Autodesk Inventor part; units mm, degrees
ref_plane "YZ Plane" through (0, 0, 0) normal (1, 0, 0) x (0, 1, 0)
ref_plane "XZ Plane" through (0, 0, 0) normal (0, 1, 0) x (-1, 0, 0)
ref_plane "XY Plane" through (0, 0, 0) normal (0, 0, 1) x (1, 0, 0)
sketch "Skizze1" plane through (0, 0, 0) normal (0, 0, 1) x (1, 0, 0)
  circle A0 centre (0, 0) radius 4.95
  circle A1 centre (-130, 0) radius 4.95
  circle A2 centre (130, 0) radius 4.95
  dimension "d0" = 9.9
  dimension "d1" = 9.9
  dimension "d2" = 130
  dimension "d3" = 9.9
  dimension "d4" = 130
extrude "Extrusion1" add sketch "Skizze1" along normal blind 10
sketch "Skizze2" plane through (0, 0, 0) normal (0, 0, -1) x (-1, 0, 0)
  line L0 (132.5, -10) -> (-132.5, -10)
  line L1 (-140, -2.5) -> (-140, 2.5)
  line L2 (-132.5, 10) -> (132.5, 10)
  line L3 (140, 2.5) -> (140, -2.5)
  arc A0 (132.5, -10) -> (140, -2.5) centre (132.5, -2.5) ccw
  arc A1 (140, 2.5) -> (132.5, 10) centre (132.5, 2.5) ccw
  arc A2 (-132.5, 10) -> (-140, 2.5) centre (-132.5, 2.5) ccw
  arc A3 (-140, -2.5) -> (-132.5, -10) centre (-132.5, -2.5) ccw
  point P0 (0, 0)
  point P1 (140, -10)
  point P2 (-140, -10)
  point P3 (140, 10)
  dimension "d7" = 20
  dimension "d8" = 280
  dimension "d9" = 140
  dimension "d10" = 7.5
  dimension "d11" = 10
extrude "Extrusion2" add sketch "Skizze2" along normal blind 10
sketch "Skizze3" plane through (0, 0, 10) normal (0, 0, 1) x (1, 0, 0)
  circle A0 centre (0, 0) radius 7.5
  circle A1 centre (130, 0) radius 7.5
  circle A2 centre (-130, 0) radius 4.95
  circle A3 centre (-130, 0) radius 7.5
  dimension "d14" = 15
  dimension "d15" = 15
  dimension "d16" = 130
  dimension "d17" = 0
  dimension "d18" = 15
extrude "Extrusion3" add sketch "Skizze3" along normal blind 5 contours A0 | A1 | A2 | A3
properties part number "Lenkung_hinten_verbindung"
The listing builds one solid part. Answer for the finished solid, in the listing's coordinates (mm). A direction names the side the tool comes from. Give positions to 0.01 mm unless a question says otherwise; leave off trailing zeros. Order: outer loops, then holes, each group sorted by start corner. A loop starts at its lowest first (then second) coordinate and runs counter-clockwise, first axis right, second up.
Item 1: For a pull along Z with two mould halves and no side action, classify faces 1 (the face through (-130, 0, 15)), 2 (the face through (132, -5, 10)), 3 (the face through (137.861, 7.745, -4.93)) as pulls with the +Z half, pulls with the -Z half, needs draft (parallel to the pull), parting line crosses it, or undercut.
From the geometry:
face 1: pulls with the +Z half
face 2: undercut
face 3: needs draft
Item 2: The part is cut by section A-A, the plane y = 0. Give the vertices of the cut face in (x, z), and give its area (3 significant figures).
From the geometry:
outline: (-140, -10) - (140, -10) - (140, 0) - (134.95, 0) - (134.95, 10) - (137.5, 10) - (137.5, 15) - (122.5, 15) - (122.5, 10) - (125.05, 10) - (125.05, 0) - (4.95, 0) - (4.95, 10) - (7.5, 10) - (7.5, 15) - (-7.5, 15) - (-7.5, 10) - (-4.95, 10) - (-4.95, 0) - (-125.05, 0) - (-125.05, 10) - (-122.5, 10) - (-122.5, 15) - (-137.5, 15) - (-137.5, 10) - (-134.95, 10) - (-134.95, 0) - (-140, 0) - close
area: 3,320 mm2
Item 3: The part is cut by section B-B, the plane x = 0. Give the vertices of the cut face in (y, z).
From the geometry:
outline: (-10, -10) - (10, -10) - (10, 0) - (4.95, 0) - (4.95, 10) - (7.5, 10) - (7.5, 15) - (-7.5, 15) - (-7.5, 10) - (-4.95, 10) - (-4.95, 0) - (-10, 0) - close
Item 4: Which of the six approach directions +Z, -Z, +X, -X, +Y, -Y give full straight-line access (tool end or side, diameter ignored) to faces 4 (the face through (2, 0, -10)), 5 (the face through (-7.493, -0.33, 12.465)), 6 (the face through (-128, -5, 10))?
From the geometry:
face 4: -Z, +X, -X, +Y, -Y
face 5: +Z
face 6: none
Item 5: Find the intervals of material crossed by probe 1 along X at (y, z) = (-1.25, 5); probe 2 along X at (y, z) = (-6.5, 13.25); probe 3 along Z at (x, y) = (-69, -5.75), in increasing order.
From the geometry:
probe 1: x = -134.79 to -125.21, -4.79 to 4.79, 125.21 to 134.79
probe 2: x = -133.74 to -126.26, -3.74 to 3.74, 126.26 to 133.74
probe 3: z = -10 to 0
Item 6: The part is cut by section C-C, the plane x = -78. Give the vertices of the cut face in (y, z), and give its area (3 significant figures).
From the geometry:
outline: (-10, -10) - (10, -10) - (10, 0) - (-10, 0) - close
area: 200 mm2
Item 7: Given pin 1 Ø10 at (x, y) = (-15, 4) entering from +Z; pin 2 Ø3 at (y, z) = (-4, 0.5) entering from +X, each flat-ended and moving along its own axis, determine where each tip first touches the part or whether it passes through.
From the geometry:
pin 1: stops at z = 0
pin 2: stops at x = 140
